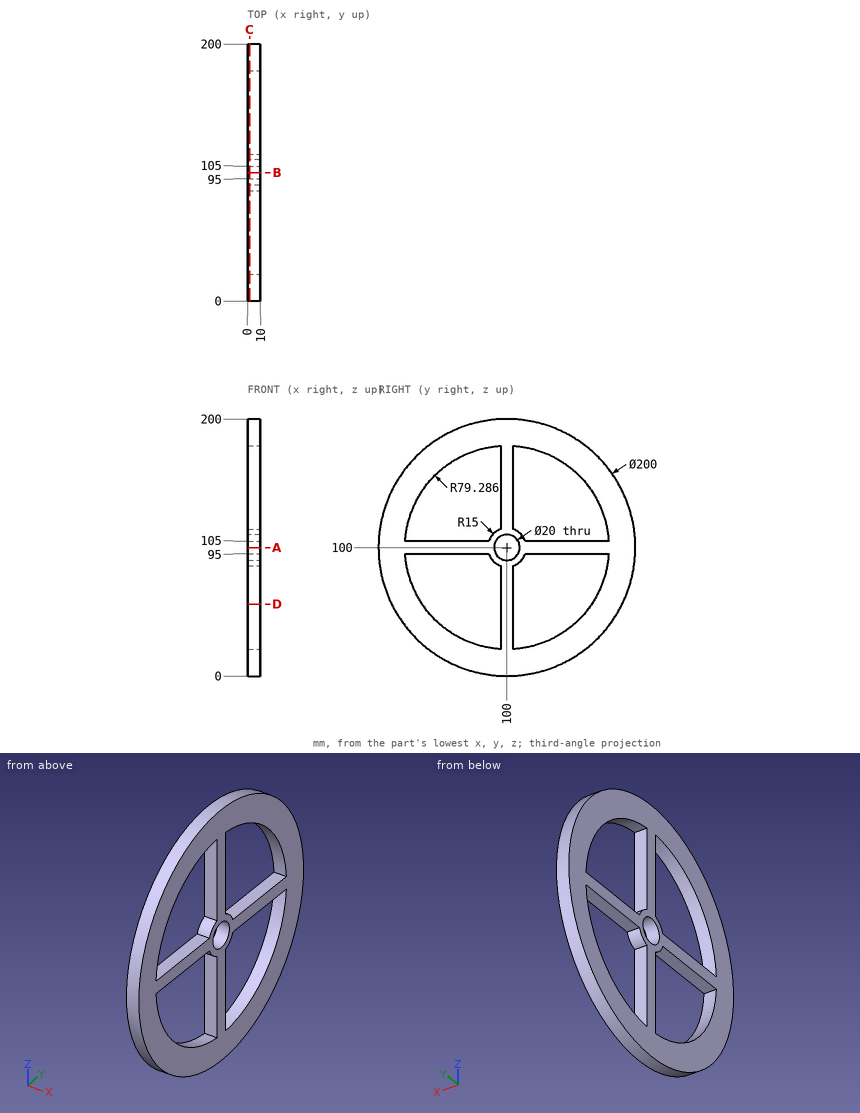
Print and shaded views of the part. All mm, measured from the part's lowest x, y and z. Coordinates: 2 decimals unless noted, no trailing zeros. Order: outer loops, then holes, each group sorted by start corner. A loop starts at its lowest first (then second) coordinate and runs counter-clockwise, first axis right, second up.
Item 1: Saw through at C-C on x = 1.5. List the corners of the cut face in (y, z).
Filled in:
outline: circle Ø200 at (100, 100); hole (20.87, 95) arc R79.29 ccw to (95, 20.87) - (95, 85.86) arc R15 cw to (85.86, 95) - close; hole (20.87, 105) - (85.86, 105) arc R15 cw to (95, 114.14) - (95, 179.13) arc R79.29 ccw to start; hole circle Ø20 at (100, 100); hole (105, 20.87) arc R79.29 ccw to (179.13, 95) - (114.14, 95) arc R15 cw to (105, 85.86) - close; hole (105, 114.14) arc R15 cw to (114.14, 105) - (179.13, 105) arc R79.29 ccw to (105, 179.13) - close
Item 2: Saw through at A-A on z = 100. List the corners of the cut face in (x, y).
Filled in:
outline: (0, 0) - (10, 0) - (10, 90) - (0, 90) - close; (0, 110) - (10, 110) - (10, 200) - (0, 200) - close
Item 3: Drop flat-ended pins along their axis: pin 1 Ø5 at (x, y) = (4.5, 41) entering from -Z; pin 2 Ø3 at (x, y) = (3, 139) entering from +Z; pin 3 Ø3 at (x, z) = (4.5, 81) entering from +Y. Give the stop position or say it passes through.
Filled in:
pin 1: stops at z = 17.49
pin 2: stops at z = 192.7
pin 3: stops at y = 198.46
Item 4: Saw through at D-D on z = 56. List the corners of the cut face in (x, y), then the cut area to 3 significant figures.
Filled in:
outline: (0, 10.2) - (10, 10.2) - (10, 34.04) - (0, 34.04) - close; (0, 95) - (10, 95) - (10, 105) - (0, 105) - close; (0, 165.96) - (10, 165.96) - (10, 189.8) - (0, 189.8) - close
area: 577 mm2
Item 5: Drill centre lines: L1, parallel to Y at x = 8.75, z = 59.5; L2, parallel to Z at x = 3.5, y = 118 (1 decimal); L3, parallel to Z at x = 8.75, y = 28 (1 decimal). Where is each one in solid material? Low to high.
Filled in:
L1: y = 8.57 to 31.84, 95 to 105, 168.16 to 191.43
L2: z = 1.6 to 22.8, 95 to 105, 177.2 to 198.4
L3: z = 30.6 to 66.8, 95 to 105, 133.2 to 169.4
